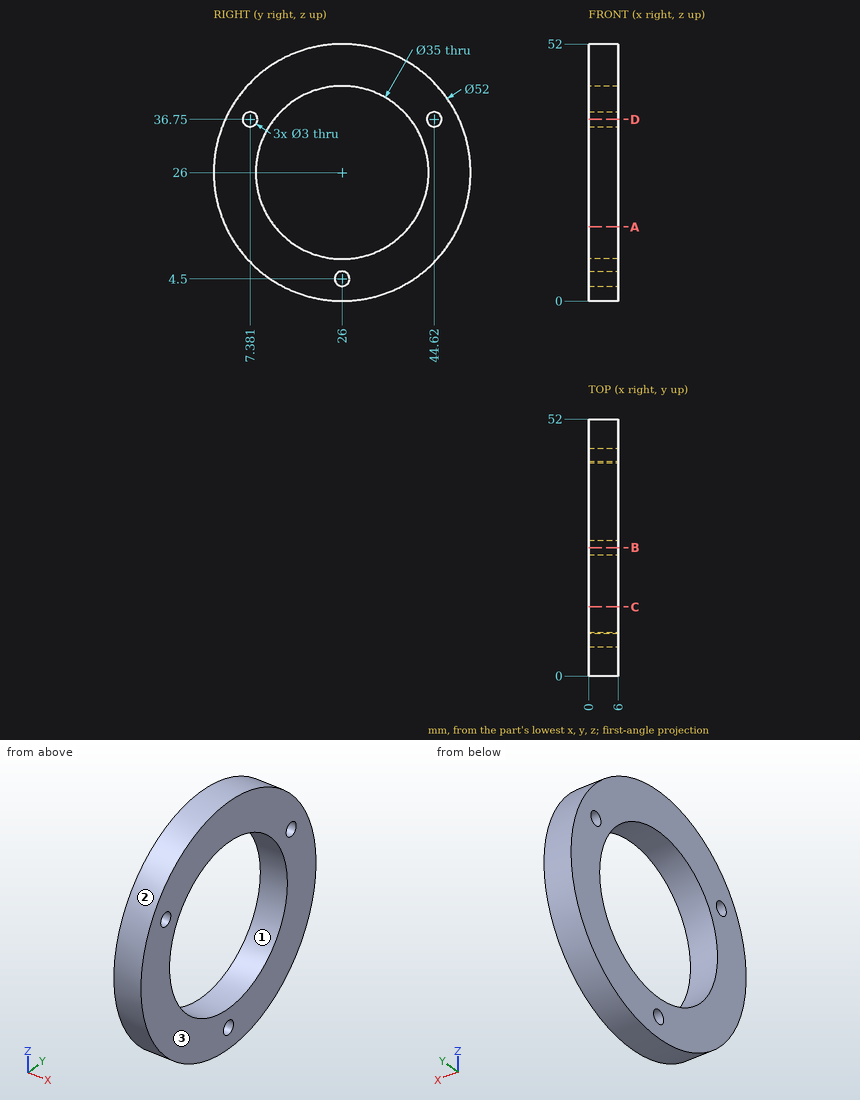
Geometry: see drawing. Coordinates: mm, zero at the bounding-box minimum. Give positions to 0.01 mm unless a question says otherwise; leave off trailing zeros. Loops run counter-clockwise (first coordinate to the right, second up) from the corner with the lowest first, then second, coordinate; pieces in that order, holes last. Notation, with made-up numbers: M 40.5,22 L 57.5,22 A13 cw 57.5,44 Z; hole C -12,1.25 d11. An arc over 180 degrees is marked long. Answer as CSV lines item,"result". Start each with the question number.
1. Section D-D on z = 36.75. Return loops of the section in (x, y).
2. Section B-B on y = 26. Return loops of the section in (x, z).
3. Pull-direction query (Y, two-part tool) for the marked faces 1, 2 and 3; classes: released by +Y, released by -Y, zero draft, split by the parting line, or undercut.
4. Section C-C on y = 14. Return loops of the section in (x, z) (1 decimal), plus the area to 3 significant figures.
5. Pin query (flat end, axial travel): P1, Ø5, axis at y = 44.62, z = 36.75, coming from the +X side; P2, Ø2.5, axis at y = 7.38, z = 36.75, coming from the -X side; P3, Ø3, axis at x = 1, y = 23, coming from the -Z side. Return the tip coordinate at first contact, or that it passes through.
6. Section A-A on z = 15. Return loops of the section in (x, y).
7. Line query: L1, parallel to Z at x = 3.1, y = 26; L2, parallel to Y at x = 2.1, z = 36.75 (1 decimal); L3, parallel to Z at x = 3.8, y = 25. Output: solid intervals per line, ascending.
Computed values:
1,outline,"M 0,2.33 L 6,2.33 L 6,5.88 L 0,5.88 Z; M 0,8.88 L 6,8.88 L 6,12.19 L 0,12.19 Z; M 0,39.81 L 6,39.81 L 6,43.12 L 0,43.12 Z; M 0,46.12 L 6,46.12 L 6,49.67 L 0,49.67 Z"
2,outline,"M 0,0 L 6,0 L 6,3 L 0,3 Z; M 0,6 L 6,6 L 6,8.5 L 0,8.5 Z; M 0,43.5 L 6,43.5 L 6,52 L 0,52 Z"
3,face 1,"undercut"
3,face 2,"split by the parting line"
3,face 3,"zero draft"
4,outline,"M 0,2.9 L 6,2.9 L 6,13.3 L 0,13.3 Z; M 0,38.7 L 6,38.7 L 6,49.1 L 0,49.1 Z"
4,area,"124 mm²"
5,P1,"stops at x = 6"
5,P2,"passes through"
5,P3,"stops at z = 0.04"
6,outline,"M 0,2.44 L 6,2.44 L 6,12.39 L 0,12.39 Z; M 0,39.61 L 6,39.61 L 6,49.56 L 0,49.56 Z"
7,L1,"z = 0 to 3, 6 to 8.5, 43.5 to 52"
7,L2,"y = 2.3 to 5.9, 8.9 to 12.2, 39.8 to 43.1, 46.1 to 49.7"
7,L3,"z = 0.02 to 3.38, 5.62 to 8.53, 43.47 to 51.98"
